Verification items for this drawing (mm, ordinates from the low corner). A direction names the side the tool comes from. Round coordinates to 2 decimals unless told otherwise and drop trailing zeros. Order: outer loops, then holes, each group sorted by start corner. A loop starts at its lowest first (then second) coordinate and runs counter-clockwise, first axis right, second up. Notation, with made-up numbers: (20.5, 18) -> (60.5, 18) arc R20 ccw to (60.5, 41) -> close; hole circle Ø5 at (-1.5, 28). An arc over 180 degrees is marked (long way). Return JSON: item names as keys, results as strings. Group by question number.
Item 1: Scan lines: probe 1 along X at (y, z) = (0.8, 3.81); probe 2 along X at (y, z) = (8.25, 4.75); probe 3 along Z at (x, y) = (3.81, 0.65). Record each from-to range of solid material in increasing order. Write a range as from..to.
Item 2: Sectioned sample at D-D on z = 6. Record the cut outline in (x, y), plus the area to 3 significant figures.
Item 3: Depth check by flat-ended pin: pin 1 Ø2 at (x, z) = (17, 4.5) entering from -Y; pin 2 Ø2 at (x, z) = (30.53, 3.81) entering from +Y; pin 3 Ø1 at (y, z) = (9.5, 5) entering from +X; pin 4 Ø4 at (y, z) = (11.5, 2.5) entering from -X. Enter the tip coordinate at first touch or a pass-through.
Item 4: Sectioned sample at B-B on z = 3.81. Record the cut outline in (x, y).
Item 5: Sectioned sample at A-A on x = 30.53. Record the cut outline in (y, z), plus the area to 3 significant figures.
Item 6: Access from +Z, -Z, +X, -X, +Y, -Y to the whole of each face (thin tool, end or side, straight path). Record for the marked faces 1, 2 and 3.
Item 7: Sectioned sample at C-C on y = 6.25. Record the cut outline in (x, z).
Item 8: Draft check along X on the marked faces 4, 5, 6 and 7. Enter one of: pulls with the +X half, pulls with the -X half, needs draft (parallel to the pull), parting line crosses it, or undercut.
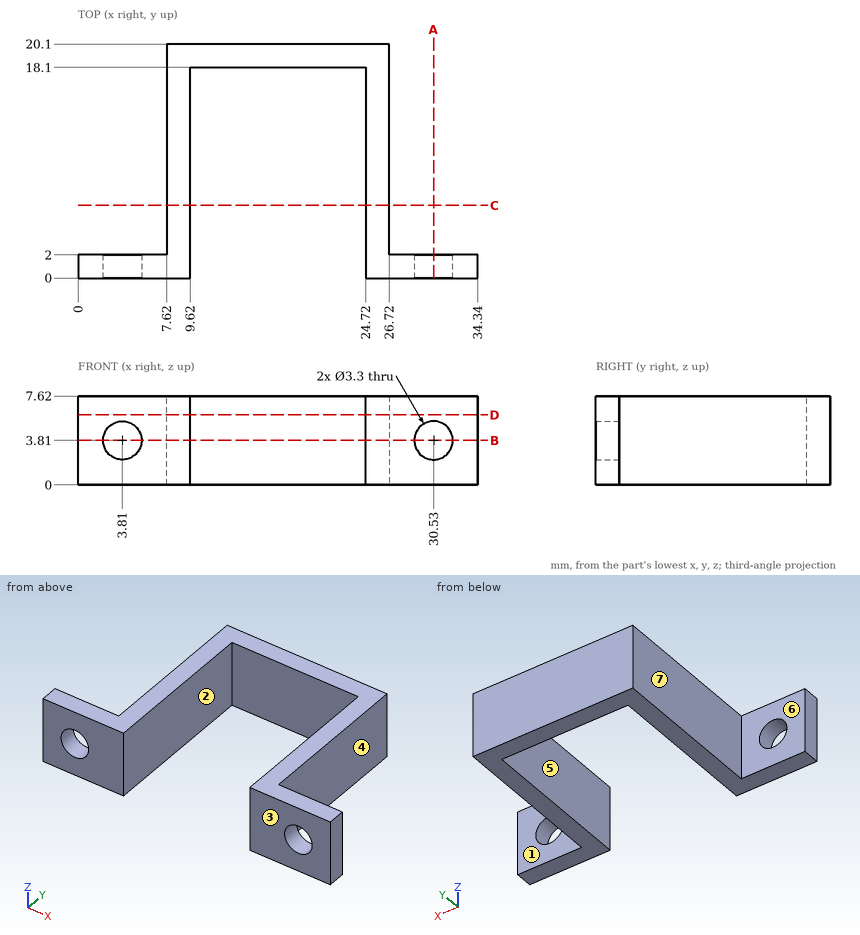
Recorded:
{
 "1": {"probe 1": "0..2.16, 5.46..9.62, 24.72..28.88, 32.18..34.34", "probe 2": "7.62..9.62, 24.72..26.72", "probe 3": "0..2.16, 5.46..7.62"},
 "2": {"outline": "(0, 0) -> (9.62, 0) -> (9.62, 18.1) -> (24.72, 18.1) -> (24.72, 0) -> (34.34, 0) -> (34.34, 2) -> (26.72, 2) -> (26.72, 20.1) -> (7.62, 20.1) -> (7.62, 2) -> (0, 2) -> close", "area": "141 mm²"},
 "3": {"pin 1": "y = 18.1", "pin 2": "through", "pin 3": "x = 26.72", "pin 4": "x = 7.62"},
 "4": {"outline": "(0, 0) -> (2.16, 0) -> (2.16, 2) -> (0, 2) -> close; (5.46, 0) -> (9.62, 0) -> (9.62, 18.1) -> (24.72, 18.1) -> (24.72, 0) -> (28.88, 0) -> (28.88, 2) -> (26.72, 2) -> (26.72, 20.1) -> (7.62, 20.1) -> (7.62, 2) -> (5.46, 2) -> close; (32.18, 0) -> (34.34, 0) -> (34.34, 2) -> (32.18, 2) -> close"},
 "5": {"outline": "(0, 0) -> (2, 0) -> (2, 2.16) -> (0, 2.16) -> close; (0, 5.46) -> (2, 5.46) -> (2, 7.62) -> (0, 7.62) -> close", "area": "8.64 mm²"},
 "6": {"face 1": "+Z, -Z, +X, +Y", "face 2": "+Z, -Z, -Y", "face 3": "+Z, -Z, +X, -X, -Y"},
 "7": {"outline": "(7.62, 0) -> (9.62, 0) -> (9.62, 7.62) -> (7.62, 7.62) -> close; (24.72, 0) -> (26.72, 0) -> (26.72, 7.62) -> (24.72, 7.62) -> close"},
 "8": {"face 4": "pulls with the +X half", "face 5": "undercut", "face 6": "needs draft", "face 7": "pulls with the -X half"}
}
